Part model, mm, in its own coordinate system. A direction names the side the tool comes from. Round coordinates to 2 decimals unless told otherwise and drop trailing zeros. Loops run counter-clockwise (first coordinate to the right, second up) from the corner with the lowest first, then second, coordinate; pieces in that order, holes last.
(1) Cut at B-B on x = 44. List the corners of the cut face in (y, z).
(2) Cut at D-D on x = 115.5. List the corners of the cut face in (y, z), then the cut area to 4 significant figures.
(3) Tool access for faces 5 (the face through (3, -1.85, 68)), 6 (the face through (63.75, 1, 82)), 7 (the face through (2, -4, 51.58)), 8 (the face through (11.6, -5, 68)): list every direction of +Z, -Z, +X, -X, +Y, -Y with a clear straight run to the whole face (end or side of a thin tool).
(4) Probe probe 1 along X at (y, z) = (-2, 61); probe 2 along X at (y, z) = (0.5, 68); probe 3 along Z at (x, y) = (41, 1.25). List the from-to ranges inside material, lowest first.
(5) Cut at A-A on z = 27. List the corners of the cut face in (x, y), then the cut area to 3 significant figures.
(6) Cut at C-C on z = 63. List the corners of the cut face in (x, y), then the cut area to 3 significant figures.
(7) Flat gauge pins, fed straight in: pin 1 (1.2 mm diameter, centred on y = -4.5, z = 60.5, fed in from +X); pin 2 (1.7 mm diameter, centred on x = 2, y = -4, fed in from -Z); pin 3 (4 mm diameter, centred on x = 38, z = 78.5, fed in from -Y). Where does each tip first touch, or does it go through?
(8) Mould opens along Z. For faces 1 (the face through (13, -4, 51.58)), 2 (the face through (64, 2.8, 4)), 3 (the face through (63.75, 1, 8)), 4 (the face through (48.1, 0.5, 90)) say: +Z half, -Z half, draft (parallel to the pull), parting line (faces both ways), or undercut.
Autodesk Inventor part; units mm, degrees
ref_plane "YZ Plane" through (0, 0, 0) normal (1, 0, 0) x (0, 1, 0)
ref_plane "XZ Plane" through (0, 0, 0) normal (0, 1, 0) x (-1, 0, 0)
ref_plane "XY Plane" through (0, 0, 0) normal (0, 0, 1) x (1, 0, 0)
sketch "Sketch1" plane through (0, 0, 0) normal (0, 0, 1) x (1, 0, 0)
  line L0 (0, 0) -> (126.5, 0)
  line L1 (126.5, 0) -> (126.5, 2.8)
  line L2 (126.5, 2.8) -> (0, 2.8)
  line L3 (0, 2.8) -> (0, 0)
  dimension "d0" = 126.5
  dimension "d1" = 2.8
extrude "Extrusion1" add sketch "Sketch1" along normal blind 90
sketch "Sketch2" plane through (0, 0, 90) normal (0, 0, 1) x (1, 0, 0)
  line L0 (126.5, 0) -> (126.5, 2.8)
  line L1 (0, 2.8) -> (0, 0)
  line L2 (126.5, 0.15) -> (127.2, 0.15)
  line L3 (127.2, 0.15) -> (127.2, 1.55)
  line L4 (127.2, 1.55) -> (126.5, 1.55)
  line L5 (126.5, 1.55) -> (126.5, 0.15)
  line L6 (0, 0.15) -> (-0.7, 0.15)
  line L7 (-0.7, 0.15) -> (-0.7, 1.55)
  line L8 (-0.7, 1.55) -> (0, 1.55)
  line L9 (0, 1.55) -> (0, 0.15)
  line L10 (126.5, 2.8) -> (0, 2.8)
  dimension "d4" = 0.7
  dimension "d5" = 1.4
  dimension "d6" = 0.7
  dimension "d7" = 1.4
  dimension "d17" = 1.25
  dimension "d18" = 1.25
extrude "Extrusion2" add sketch "Sketch2" against normal blind 85
sketch "Sketch3" plane through (0, 0, 0) normal (0, -1, 0) x (1, 0, 0)
  line L0 (0, 90) -> (126.5, 90)
  line L1 (0, 0) -> (0, 90)
  line L2 (0.6, 90) -> (15.1, 90)
  line L3 (15.1, 90) -> (15.1, 84.58)
  line L4 (15.1, 84.58) -> (0.6, 84.58)
  line L5 (0.6, 84.58) -> (0.6, 90)
  dimension "d12" = 14.5
  dimension "d13" = 5.42
  dimension "d14" = 0.6
extrude "Extrusion3" add sketch "Sketch3" along normal blind 5.72
sketch "Sketch4" plane through (0, 0, 0) normal (0, -1, 0) x (1, 0, 0)
  line L0 (15.1, 90) -> (15.1, 84.58)
  line L1 (15.1, 84.58) -> (0.6, 84.58)
  line L2 (0.6, 84.58) -> (0.6, 90)
  line L3 (0, 90) -> (0.6, 90)
  line L4 (0, 0) -> (0, 90)
  line L5 (0, 0) -> (126.5, 0)
  line L6 (126.5, 0) -> (126.5, 90)
  line L7 (15.1, 90) -> (126.5, 90)
extrude "Extrusion4" cut sketch "Sketch4" against normal blind 0.15
sketch "Sketch5" plane through (0, 0.15, 0) normal (0, -1, 0) x (1, 0, 0)
  line L0 (0.6, 84.58) -> (15.1, 84.58)
  line L1 (0.6, 84.58) -> (2.6, 84.58)
  line L2 (2.6, 84.58) -> (2.6, 51.58)
  line L3 (2.6, 51.58) -> (0.6, 51.58)
  line L4 (0.6, 51.58) -> (0.6, 84.58)
  line L5 (15.1, 84.58) -> (13.1, 84.58)
  line L6 (13.1, 84.58) -> (13.1, 51.58)
  line L7 (13.1, 51.58) -> (15.1, 51.58)
  line L8 (15.1, 51.58) -> (15.1, 84.58)
  dimension "d21" = 33
  dimension "d22" = 2
  dimension "d23" = 2
  dimension "d24" = 10.5
extrude "Extrusion5" add sketch "Sketch5" along normal blind 6
sketch "Sketch6" plane through (2.6, 0.15, 51.58) normal (0, 0, -1) x (-1, 0, 0)
  line L0 (0, 0) -> (0, -6)
  line L1 (2, -6) -> (0, -6)
  line L2 (0, -2) -> (-1.5, -2)
  line L3 (-1.5, -2) -> (-1.5, 0)
  line L4 (-1.5, 0) -> (0, 0)
  line L5 (0, 0) -> (0, -2)
  point P0 (2.6, -0.15)
  dimension "d27" = 4
  dimension "d28" = 2
  dimension "d29" = 1.5
extrude "Extrusion6" add sketch "Sketch6" against normal blind 33
sketch "Sketch7" plane through (2.6, -5.85, 51.58) normal (0, 0, -1) x (-1, 0, 0)
  line L0 (0, 4) -> (1.65, 4)
  line L1 (1.65, 4) -> (1.65, 2.4)
  line L2 (1.65, 2.4) -> (0, 2.4)
  line L3 (0, 2.4) -> (0, 4)
  point P0 (2.6, 5.85)
  dimension "d32" = 1.65
  dimension "d33" = 1.6
extrude "Extrusion7" cut sketch "Sketch7" against normal blind 33
sketch "Sketch8" plane through (15.1, 0.15, 51.58) normal (0, 0, -1) x (-1, 0, 0)
  line L0 (2, 0) -> (3.5, 0)
  line L1 (3.5, 0) -> (3.5, -2)
  line L2 (3.5, -2) -> (2, -2)
  line L3 (2, -2) -> (2, 0)
  point P0 (15.1, -0.15)
  dimension "d36" = 1.5
  dimension "d37" = 2
extrude "Extrusion8" add sketch "Sketch8" against normal blind 33
sketch "Sketch9" plane through (15.1, -5.85, 51.58) normal (0, 0, -1) x (-1, 0, 0)
  line L0 (2, 4) -> (0.35, 4)
  line L1 (0.35, 4) -> (0.35, 2.4)
  line L2 (0.35, 2.4) -> (2, 2.4)
  line L3 (2, 2.4) -> (2, 4)
  point P0 (15.1, 5.85)
  dimension "d40" = 1.65
  dimension "d41" = 1.6
extrude "Extrusion9" cut sketch "Sketch9" against normal blind 33
sketch "Sketch10" plane through (13.1, -5.85, 51.58) normal (-1, 0, 0) x (0, 0, 1)
  line L0 (33, 2.4) -> (0, 2.4)
  line L1 (0, 2.4) -> (0, 0)
  line L2 (33, 0) -> (0, 0)
  line L3 (33, 0.13) -> (33, 0)
  line L4 (33, 2.4) -> (33, 0.13)
  point P0 (-51.58, 5.85)
extrude "Extrusion10" add sketch "Sketch10" along normal blind 1.5
sketch "Sketch11" plane through (2.6, -5.85, 84.58) normal (1, 0, 0) x (0, 0, -1)
  line L0 (33, 2.4) -> (0, 2.4)
  line L1 (0, 0.13) -> (0, 2.4)
  line L2 (0, 0.13) -> (0, 0)
  line L3 (33, 0) -> (0, 0)
  line L4 (33, 2.4) -> (33, 0)
  point P0 (84.58, 5.85)
extrude "Extrusion11" add sketch "Sketch11" along normal blind 1.5
sketch "Sketch12" plane through (0, 2.8, 0) normal (0, 1, 0) x (1, 0, 0)
  line L0 (18.25, -10) -> (108.25, -10)
  line L1 (108.25, -10) -> (108.25, -80)
  line L2 (108.25, -80) -> (18.25, -80)
  line L3 (18.25, -80) -> (18.25, -10)
  line L4 (126.5, 0) -> (0, 0)
  line L5 (0, 0) -> (0, -90)
  line L6 (126.5, -90) -> (0, -90)
  line L7 (126.5, 0) -> (126.5, -90)
  line L8 (47.32, -80) -> (63.75, -80)
  line L9 (63.75, -80) -> (63.75, -85)
  line L10 (63.75, -85) -> (47.32, -85)
  line L11 (47.32, -85) -> (47.32, -80)
  line L12 (47.32, -10) -> (63.75, -10)
  line L13 (63.75, -10) -> (63.75, -5)
  line L14 (63.75, -5) -> (47.32, -5)
  line L15 (47.32, -5) -> (47.32, -10)
  dimension "d51" = 90
  dimension "d52" = 70
  dimension "d55" = 18.25
  dimension "d56" = 18.25
  dimension "d57" = 10
  dimension "d58" = 10
  dimension "d59" = 16.43
  dimension "d60" = 5
  dimension "d61" = 29.07
  dimension "d67" = 5
  dimension "d68" = 29.07
extrude "Extrusion13" cut sketch "Sketch12" against normal up to next contours L0 L1 L2 L3 | L15 L14 L13 L0 | L2 L9 L10 L11
chamfer "Chamfer1" distance 1.2 angle 60 1 edges at (47.32, 2.8, 82.5) measured on face at (6.0833, 2.8, 56.6667)
chamfer "Chamfer2" distance 1.2 angle 60 1 edges at (47.32, 2.8, 7.5) measured on face at (6.0833, 2.8, 56.6667)
properties part number "Bovenplaat Frame 2.3"
Final values:
1. outline: (0.15, 0) - (2.8, 0) - (2.8, 10) - (0.15, 10) - close; (0.15, 80) - (2.8, 80) - (2.8, 90) - (0.15, 90) - close
2. outline: (0.15, 0) - (2.8, 0) - (2.8, 90) - (0.15, 90) - close
2. area: 238.5 mm2
3. face 5: -Z
3. face 6: +Y, -Y
3. face 7: -Z, +X, -X, -Y
3. face 8: -Z, -Y
4. probe 1: x = 0.6 to 0.95, 14.75 to 15.1
4. probe 2: x = -0.7 to 18.25, 108.25 to 127.2
4. probe 3: z = 0 to 10, 80 to 90
5. outline: (-0.7, 0.15) - (18.25, 0.15) - (18.25, 2.8) - (0, 2.8) - (0, 1.55) - (-0.7, 1.55) - close; (108.25, 0.15) - (127.2, 0.15) - (127.2, 1.55) - (126.5, 1.55) - (126.5, 2.8) - (108.25, 2.8) - close
5. area: 98.7 mm2
6. outline: (-0.7, 0.15) - (0.6, 0.15) - (0.6, -5.85) - (4.1, -5.85) - (4.1, -3.45) - (0.95, -3.45) - (0.95, -1.85) - (4.1, -1.85) - (4.1, 0.15) - (11.6, 0.15) - (11.6, -1.85) - (14.75, -1.85) - (14.75, -3.45) - (11.6, -3.45) - (11.6, -5.85) - (15.1, -5.85) - (15.1, 0.15) - (18.25, 0.15) - (18.25, 2.8) - (0, 2.8) - (0, 1.55) - (-0.7, 1.55) - close; (108.25, 0.15) - (127.2, 0.15) - (127.2, 1.55) - (126.5, 1.55) - (126.5, 2.8) - (108.25, 2.8) - close
6. area: 131 mm2
7. pin 1: stops at x = 15.1
7. pin 2: stops at z = 51.58
7. pin 3: stops at y = 0.15
8. face 1: -Z half
8. face 2: draft
8. face 3: undercut
8. face 4: +Z half
